```python
from build123d import *

# Parameters (mm, degrees)
F1_DEPTH = 8
F0_W     = 11
F0_H     = 20
F0_W_2   = 7
F0_H_2   = 16
F2_DEPTH = 4


with BuildPart() as f1:
    # F0 (on Top) → F1 (new body)
    with BuildSketch(Plane.XY):
        Polygon((11, -46.5), (11, 46.5), (0, 46.5), (-11, 46.5), (-11, -46.5), align=None)
        Polygon((8.25, -21.494463), (8.25, -25.494463), (3.5, -25.494463), (3.5, -41.494463), (-3.5, -41.494463), (-3.5, -25.494463), (-8.25, -25.494463), (-8.25, -21.494463), (-3.5, -21.494463), (-3.5, -5.494463), (3.5, -5.494463), (3.5, -21.494463), align=None, mode=Mode.SUBTRACT)
    extrude(amount=F1_DEPTH)

    # F0 (on Top) → F2 (join)
    with BuildSketch(Plane.XY):
        with Locations((5.5, 56.5)):
            Rectangle(F0_W, F0_H)
        with Locations((0, -13.494463)):
            Rectangle(F0_W_2, F0_H_2)
        Polygon((3.5, -25.494463), (8.25, -25.494463), (8.25, -21.494463), (3.5, -21.494463), (-3.5, -21.494463), (-8.25, -21.494463), (-8.25, -25.494463), (-3.5, -25.494463), align=None)
        with Locations((0, -33.494463)):
            Rectangle(F0_W_2, F0_H_2)
        with Locations((-5.5, 56.5)):
            Rectangle(F0_W, F0_H)
    extrude(amount=F2_DEPTH)


solid = f1.part
```
The listing builds one solid part. Answer for the finished solid, in the listing's coordinates (mm). A direction names the side the tool comes from. Coordinates: 2 decimals unless noted, no trailing zeros. Write each loop counter-clockwise with the first axis right and the second up, starting at its lowest first coordinate (ties: lowest second). Pieces come first, ordered by that corner, then holes. Notation, with made-up numbers: (83, 17.5) - (97, 17.5) arc R11 cw to (97, 32.5) - close; hole circle Ø2 at (6.5, 77). An arc over 180 degrees is marked (long way). Return JSON: item names as keys, results as strings. Group by question number.
Q1. For a pull along X with two mould halves and no side action, classify faces 1 (the flat face through (0, 66.5, 2)), 2 (the flat face through (-11, 9, 4)), 3 (the flat face through (-8.25, -24, 6)) as +X half, -X half, draft (parallel to the pull), parting line (faces both ways), or undercut.
Q2. The part is cut by section D-D on x = 1. Write down the section's boundary in (y, z), and give its area (3 significant figures).
Q3. The part is cut by section B-B on x = 5.25. Write down the section's boundary in (y, z), and give its area (3 significant figures).
Q4. The part is cut by section C-C on y = -35. Write down the section's boundary in (x, z).
Q5. Which of the six approach directions +Z, -Z, +X, -X, +Y, -Y give full straight-line access (tool end or side, diameter ignored) to faces 4 (the flat face through (0, -46.5, 4)), 5 (the flat face through (0, -41.494, 6)), 6 (the flat face through (0, 57, 4))?
Q6. The part is cut by section A-A on z = 6.5. Write down the section's boundary in (x, y), and give its area (3 significant figures).
Q7. Find the intervals of material crossed by line 1 along X through (y, z) = (-21, 7.25); line 2 along Y through (x, z) = (-7.5, 6.75); line 3 along Y through (x, z) = (-2.5, 7.5), in increasing order. Write a range as [from, to].
Q8. A flat-ended cylindrical pin translates along its axis: pin 1 Ø3 at (x, z) = (1, 6) entering from +Y. Find the tip coordinate at first contact, or state that the pin passes through.
Evaluation:
{
 "1": {"face 1": "draft", "face 2": "-X half", "face 3": "undercut"},
 "2": {"outline": "(-46.5, 0) - (66.5, 0) - (66.5, 4) - (46.5, 4) - (46.5, 8) - (-5.49, 8) - (-5.49, 4) - (-41.49, 4) - (-41.49, 8) - (-46.5, 8) - close", "area": "680 mm2"},
 "3": {"outline": "(-46.5, 0) - (66.5, 0) - (66.5, 4) - (46.5, 4) - (46.5, 8) - (-21.49, 8) - (-21.49, 4) - (-25.49, 4) - (-25.49, 8) - (-46.5, 8) - close", "area": "808 mm2"},
 "4": {"outline": "(-11, 0) - (11, 0) - (11, 8) - (3.5, 8) - (3.5, 4) - (-3.5, 4) - (-3.5, 8) - (-11, 8) - close"},
 "5": {"face 4": "+Z, -Z, +X, -X, -Y", "face 5": "+Z", "face 6": "+Z, +X, -X, +Y"},
 "6": {"outline": "(-11, -46.5) - (11, -46.5) - (11, 46.5) - (-11, 46.5) - close; hole (-8.25, -25.49) - (-3.5, -25.49) - (-3.5, -41.49) - (3.5, -41.49) - (3.5, -25.49) - (8.25, -25.49) - (8.25, -21.49) - (3.5, -21.49) - (3.5, -5.49) - (-3.5, -5.49) - (-3.5, -21.49) - (-8.25, -21.49) - close", "area": "1,760 mm2"},
 "7": {"line 1": "x = [-11, -3.5], [3.5, 11]", "line 2": "y = [-46.5, -25.49], [-21.49, 46.5]", "line 3": "y = [-46.5, -41.49], [-5.49, 46.5]"},
 "8": {"pin 1": "stops at y = 46.5"}
}
